from build123d import *

# Parameters (mm, degrees)
SKETCH_W        = 12
SKETCH_H        = 77
PAD_DEPTH       = 5
PAD001_DEPTH    = 5.1
PAD002_DEPTH    = 3
SKETCH003_W     = 4
SKETCH003_H     = 105
SKETCH003_W_2   = 10
SKETCH003_H_2   = 5
PAD003_DEPTH    = 12
SKETCH004_W     = 4.6
SKETCH004_H     = 10
POCKET_DEPTH    = 2.5
POCKET001_DEPTH = 12.001
FILLET_R        = 2
CHAMFER_SIZE    = 1


with BuildPart() as part:
    # Sketch → Pad (new body)
    with BuildSketch(Plane.XZ):
        with Locations((0, 38.5)):
            Rectangle(SKETCH_W, SKETCH_H)
    extrude(amount=PAD_DEPTH)

    # Sketch001 (on Face6 of Pad) → Pad001 (join)
    with BuildSketch(Plane.XZ.offset(5)):
        with BuildLine():
            Line((-2.2, 25.05), (-2.2, 22.45))
            ThreePointArc((-2.2, 22.45), (0, 20.25), (2.2, 22.45))
            Line((2.2, 25.05), (2.2, 22.45))
            ThreePointArc((2.2, 25.05), (0, 27.25), (-2.2, 25.05))
        make_face()
        with BuildLine():
            Line((-2.2, 65.05), (-2.2, 62.45))
            ThreePointArc((-2.2, 62.45), (0, 60.25), (2.2, 62.45))
            Line((2.2, 65.05), (2.2, 62.45))
            ThreePointArc((2.2, 65.05), (0, 67.25), (-2.2, 65.05))
        make_face()
    extrude(amount=PAD001_DEPTH)

    # Sketch002 (on Face16 of Pad001) → Pad002 (join)
    with BuildSketch(Plane.XZ.offset(10.1)):
        with BuildLine():
            Line((-2.2, 25.05), (-2.2, 16.45))
            ThreePointArc((-2.2, 16.45), (0, 14.25), (2.2, 16.45))
            Line((2.2, 25.05), (2.2, 16.45))
            ThreePointArc((2.2, 25.05), (0, 27.25), (-2.2, 25.05))
        make_face()
        with BuildLine():
            Line((-2.2, 65.05), (-2.2, 56.45))
            ThreePointArc((-2.2, 56.45), (0, 54.25), (2.2, 56.45))
            Line((2.2, 65.05), (2.2, 56.45))
            ThreePointArc((2.2, 65.05), (0, 67.25), (-2.2, 65.05))
        make_face()
    extrude(amount=PAD002_DEPTH)

    # Sketch003 (on Face6 of Pad002) → Pad003 (join)
    with BuildSketch(Plane(origin=(6, 0, 0), x_dir=(0, 0, 1), z_dir=(1, 0, 0))):
        with Locations((2, -52.5)):
            Rectangle(SKETCH003_W, SKETCH003_H)
        with Locations((9, -12.5)):
            Rectangle(SKETCH003_W_2, SKETCH003_H_2)
        with Locations((9, -27.5)):
            Rectangle(SKETCH003_W_2, SKETCH003_H_2)
        with Locations((9, -42.5)):
            Rectangle(SKETCH003_W_2, SKETCH003_H_2)
        with Locations((9, -57.5)):
            Rectangle(SKETCH003_W_2, SKETCH003_H_2)
        with Locations((9, -72.5)):
            Rectangle(SKETCH003_W_2, SKETCH003_H_2)
        with Locations((9, -87.5)):
            Rectangle(SKETCH003_W_2, SKETCH003_H_2)
        with Locations((9, -102.5)):
            Rectangle(SKETCH003_W_2, SKETCH003_H_2)
    extrude(amount=-PAD003_DEPTH)

    # Sketch004 (on Face30 of Pad003) → Pocket (cut)
    with BuildSketch(Plane(origin=(0, 0, 4), x_dir=(-1, 0, 0), z_dir=(0, 0, 1))):
        with Locations((0, -5)):
            Rectangle(SKETCH004_W, SKETCH004_H)
        with Locations((0, -20)):
            Rectangle(SKETCH004_W, SKETCH004_H)
        with Locations((0, -35)):
            Rectangle(SKETCH004_W, SKETCH004_H)
        with Locations((0, -50)):
            Rectangle(SKETCH004_W, SKETCH004_H)
        with Locations((0, -65)):
            Rectangle(SKETCH004_W, SKETCH004_H)
        with Locations((0, -80)):
            Rectangle(SKETCH004_W, SKETCH004_H)
        with Locations((0, -95)):
            Rectangle(SKETCH004_W, SKETCH004_H)
    extrude(amount=-POCKET_DEPTH, mode=Mode.SUBTRACT)

    # Sketch005 (on Face5 of Pocket) → Pocket001 (cut, through all)
    with BuildSketch(Plane(origin=(6, 0, 0), x_dir=(0, 0, 1), z_dir=(1, 0, 0))):
        with BuildLine():
            ThreePointArc((74.499999, 0), (77, 2.5), (74.5, 5))
            Line((74.5, 5), (77.1, 5))
            Line((77.1, 5), (77.099999, 0))
            Line((74.499999, 0), (77.099999, 0))
        make_face()
    extrude(amount=-POCKET001_DEPTH, mode=Mode.SUBTRACT)

    # Fillet
    fillet_edges = [part.edges().sort_by_distance(p)[0] for p in [
        (0, 105, 0),
        (0, -5, 0),
        (0, 105, 14),
        (0, 100, 14),
        (0, 90, 14),
        (0, 85, 14),
        (0, 75, 14),
        (0, 70, 14),
        (0, 60, 14),
        (0, 55, 14),
        (0, 45, 14),
        (0, 40, 14),
        (0, 30, 14),
        (0, 25, 14),
        (0, 15, 14),
        (0, 10, 14),
    ]]
    fillet(fillet_edges, radius=FILLET_R)

    # Chamfer
    chamfer_edges = [part.edges().sort_by_distance(p)[0] for p in [
        (6, -5, 38.25),
        (6, -4.414214, 0.585786),
        (6, -4.267767, 76.267767),
        (6, 50, 0),
        (6, -0.732233, 76.267767),
        (6, 104.414214, 0.585786),
        (6, 0, 39.25),
        (6, 105, 7),
        (6, 5, 4),
        (6, 104.414214, 13.414214),
        (6, 10, 8),
        (6, 102.5, 14),
        (6, 10.585786, 13.414214),
        (6, 100.585786, 13.414214),
        (6, 12.5, 14),
        (6, 100, 8),
        (6, 14.414214, 13.414214),
        (6, 95, 4),
        (6, 15, 8),
        (6, 90, 8),
        (6, 20, 4),
        (6, 89.414214, 13.414214),
        (6, 25, 8),
        (6, 87.5, 14),
        (6, 25.585786, 13.414214),
        (6, 85.585786, 13.414214),
        (6, 27.5, 14),
        (6, 85, 8),
        (6, 29.414214, 13.414214),
        (6, 80, 4),
        (6, 30, 8),
        (6, 75, 8),
        (6, 35, 4),
        (6, 74.414214, 13.414214),
        (6, 40, 8),
        (6, 72.5, 14),
        (6, 40.585786, 13.414214),
        (6, 70.585786, 13.414214),
        (6, 42.5, 14),
        (6, 70, 8),
        (6, 44.414214, 13.414214),
        (6, 65, 4),
        (6, 45, 8),
        (6, 60, 8),
        (6, 50, 4),
        (6, 59.414214, 13.414214),
        (6, 55, 8),
        (6, 57.5, 14),
        (6, 55.585786, 13.414214),
        (-6, -5, 38.25),
        (-6, -4.414214, 0.585786),
        (-6, -4.267767, 76.267767),
        (-6, 50, 0),
        (-6, -0.732233, 76.267767),
        (-6, 104.414214, 0.585786),
        (-6, 0, 39.25),
        (-6, 105, 7),
        (-6, 5, 4),
        (-6, 104.414214, 13.414214),
        (-6, 10, 8),
        (-6, 102.5, 14),
        (-6, 10.585786, 13.414214),
        (-6, 100.585786, 13.414214),
        (-6, 12.5, 14),
        (-6, 100, 8),
        (-6, 14.414214, 13.414214),
        (-6, 95, 4),
        (-6, 15, 8),
        (-6, 90, 8),
        (-6, 20, 4),
        (-6, 89.414214, 13.414214),
        (-6, 25, 8),
        (-6, 87.5, 14),
        (-6, 25.585786, 13.414214),
        (-6, 85.585786, 13.414214),
        (-6, 27.5, 14),
        (-6, 85, 8),
        (-6, 29.414214, 13.414214),
        (-6, 80, 4),
        (-6, 30, 8),
        (-6, 75, 8),
        (-6, 35, 4),
        (-6, 74.414214, 13.414214),
        (-6, 40, 8),
        (-6, 72.5, 14),
        (-6, 40.585786, 13.414214),
        (-6, 70.585786, 13.414214),
        (-6, 42.5, 14),
        (-6, 70, 8),
        (-6, 44.414214, 13.414214),
        (-6, 65, 4),
        (-6, 45, 8),
        (-6, 60, 8),
        (-6, 50, 4),
        (-6, 59.414214, 13.414214),
        (-6, 55, 8),
        (-6, 57.5, 14),
        (-6, 55.585786, 13.414214),
    ]]
    chamfer(chamfer_edges, length=CHAMFER_SIZE)


solid = part.part
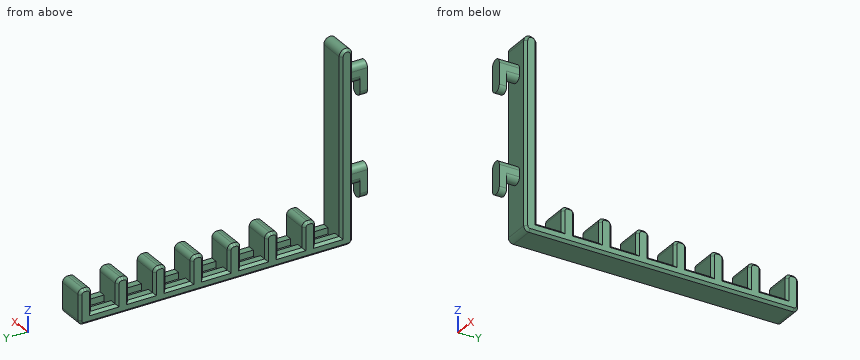
The listing builds one solid part. Answer for the finished solid, in the listing's coordinates (mm). Round coordinates to 2 decimals unless told otherwise and drop trailing zeros. Order: outer loops, then holes, each group sorted by start corner. A loop starts at its lowest first (then second) coordinate and runs counter-clockwise, first axis right, second up. Notation, with made-up numbers: (69, 89) - (89, 89) arc R32 cw to (89, 115) - close; hole circle Ø2 at (23, 59). An arc over 180 degrees is marked (long way). Write item = value, one per line. Start each with the question number.
1) Given pin 1 (3 mm diameter, centred on x = 3, z = 65, fed in from +Y); pin 2 (4 mm diameter, centred on x = 0.5, z = 46.5, fed in from -Y); pin 3 (1.4 mm diameter, centred on x = -3.5, y = 35.5, fed in from +Z), each flat-ended and moving along its own axis, determine where each tip first touches the part or whether it passes through.
2) Straight lines are drawn through the part: L1, parallel to Z at x = 0.5, y = 65.5; L2, parallel to Y at x = 1.5, z = 22; L3, parallel to Z at x = 4, y = 53.5. For each, find the intervals that lie inside material, in ascending order.
3) Section C-C, the plane z = 47 is taken. Write down the section's boundary in (x, y).
4) Section B-B, the plane y = 68.5 is taken. Write down the section's boundary in (x, z).
5) Section A-A, the plane z = 58.5 is taken. Write down the section's boundary in (x, y).
Results list:
q1.pin_1 = 0
q1.pin_2 = -5
q1.pin_3 = 4
q2.L1 = 0 to 1.5
q2.L2 = -13.1 to 0
q2.L3 = 0 to 4
q3.outline = (-6, -4) - (-5, -5) - (5, -5) - (6, -4) - (6, -1) - (5, 0) - (-5, 0) - (-6, -1) - close
q4.outline = (-6, 1) - (-5, 0) - (5, 0) - (6, 1) - (6, 3) - (5, 4) - (2.3, 4) - (2.3, 1.5) - (-2.3, 1.5) - (-2.3, 4) - (-5, 4) - (-6, 3) - close
q5.outline = (-6, -4) - (-5, -5) - (5, -5) - (6, -4) - (6, -1) - (5, 0) - (-5, 0) - (-6, -1) - close; (-2.2, -13.1) - (2.2, -13.1) - (2.2, -10.1) - (-2.2, -10.1) - close
